Drawing for the job (mm, zero at the part's lowest x, y, z). A direction names the side the tool comes from. Coordinates: 2 decimals unless noted, no trailing zeros. Write each loop counter-clockwise with the first axis right and the second up, starting at its lowest first coordinate (ties: lowest second). Pieces come first, ordered by that corner, then holes. Notation, with made-up numbers: M 20,62 L 31,62 A21 cw 31,95 Z; hole C -10,-28.5 d3. An arc over 180 degrees is marked long. Put each result on its own line as item: value. Start each with the question number.
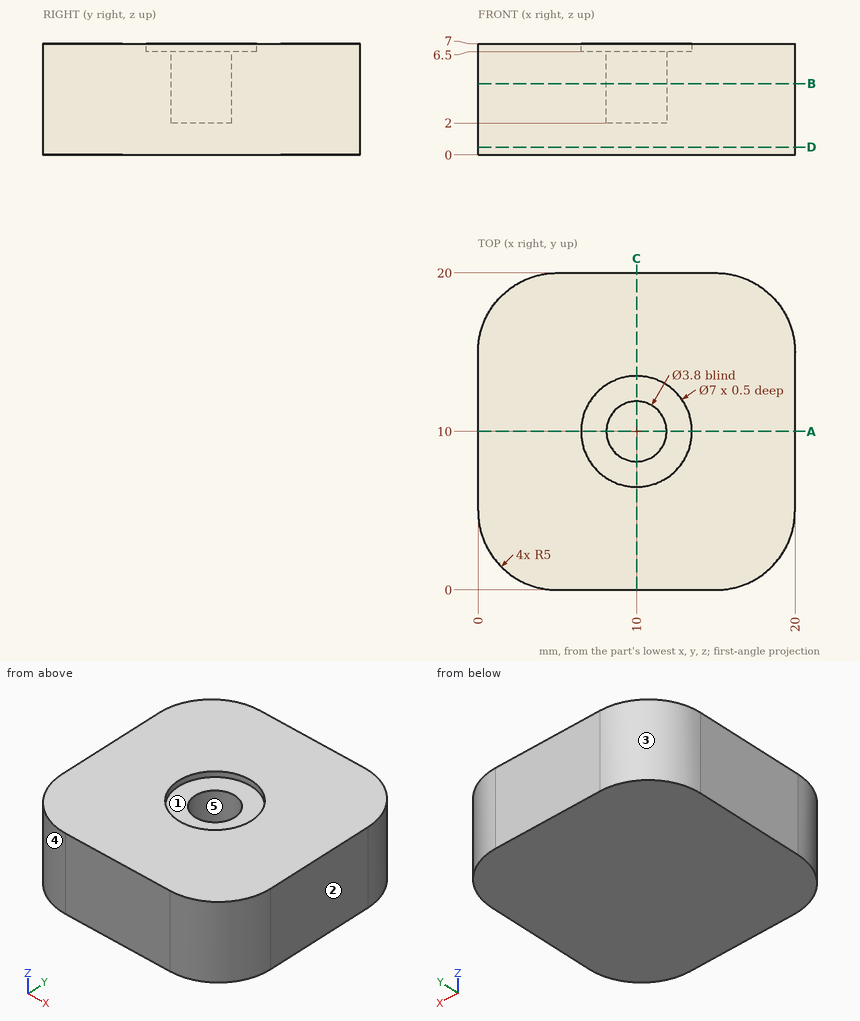
(1) Two-plate mould, pull along X, no slides. Class the marked faces 1, 2 and 3: +X half, -X half, draft (parallel to the pull), parting line (faces both ways), or undercut.
(2) Drill centre lines: line 1 (Y direction, x = 10, z = 6.8); line 2 (Y direction, x = 10, z = 4.8); line 3 (Y direction, x = 4.75, z = 3.5). Where is each one in solid material? Low to high. Write a range as [from, to].
(3) Slice it at D-D, the plane z = 0.5. Write the cut outline in (x, y), then the cut area to 3 significant figures.
(4) Drop flat-ended pins along their axis: pin 1 (5 mm diameter, centred on x = 10, y = 10, fed in from +Z); pin 2 (3 mm diameter, centred on x = 14, z = 5, fed in from -Y); pin 3 (1.9 mm diameter, centred on x = 9.5, y = 9.5, fed in from +Z); pin 4 (2 mm diameter, centred on y = 3, z = 3.5, fed in from +X). Give the stop position or say it passes through.
(5) Slice it at B-B, the plane z = 4.5. Write the cut outline in (x, y).
(6) Slice it at A-A, the plane y = 10. Write the cut outline in (x, z).
(7) Which spindle directions (+Z, -Z, +X, -X, +Y, -Y) get a long thin tool onto all of the face, cutting with end or side? Do the marked faces 4 and 5. Say none if no direction does.
Result set:
1. face 1: undercut
1. face 2: +X half
1. face 3: -X half
2. line 1: y = [0, 6.5], [13.5, 20]
2. line 2: y = [0, 8.1], [11.9, 20]
2. line 3: y = [0.01, 19.99]
3. outline: M 0,5 A5 ccw 5,0 L 15,0 A5 ccw 20,5 L 20,15 A5 ccw 15,20 L 5,20 A5 ccw 0,15 Z
3. area: 379 mm^2
4. pin 1: stops at z = 6.5
4. pin 2: stops at y = 0
4. pin 3: stops at z = 2
4. pin 4: stops at x = 19.9
5. outline: M 0,5 A5 ccw 5,0 L 15,0 A5 ccw 20,5 L 20,15 A5 ccw 15,20 L 5,20 A5 ccw 0,15 Z; hole C 10,10 d3.8
6. outline: M 0,0 L 20,0 L 20,7 L 13.5,7 L 13.5,6.5 L 11.9,6.5 L 11.9,2 L 8.1,2 L 8.1,6.5 L 6.5,6.5 L 6.5,7 L 0,7 Z
7. face 4: +Z, -Z, -X, -Y
7. face 5: +Z
